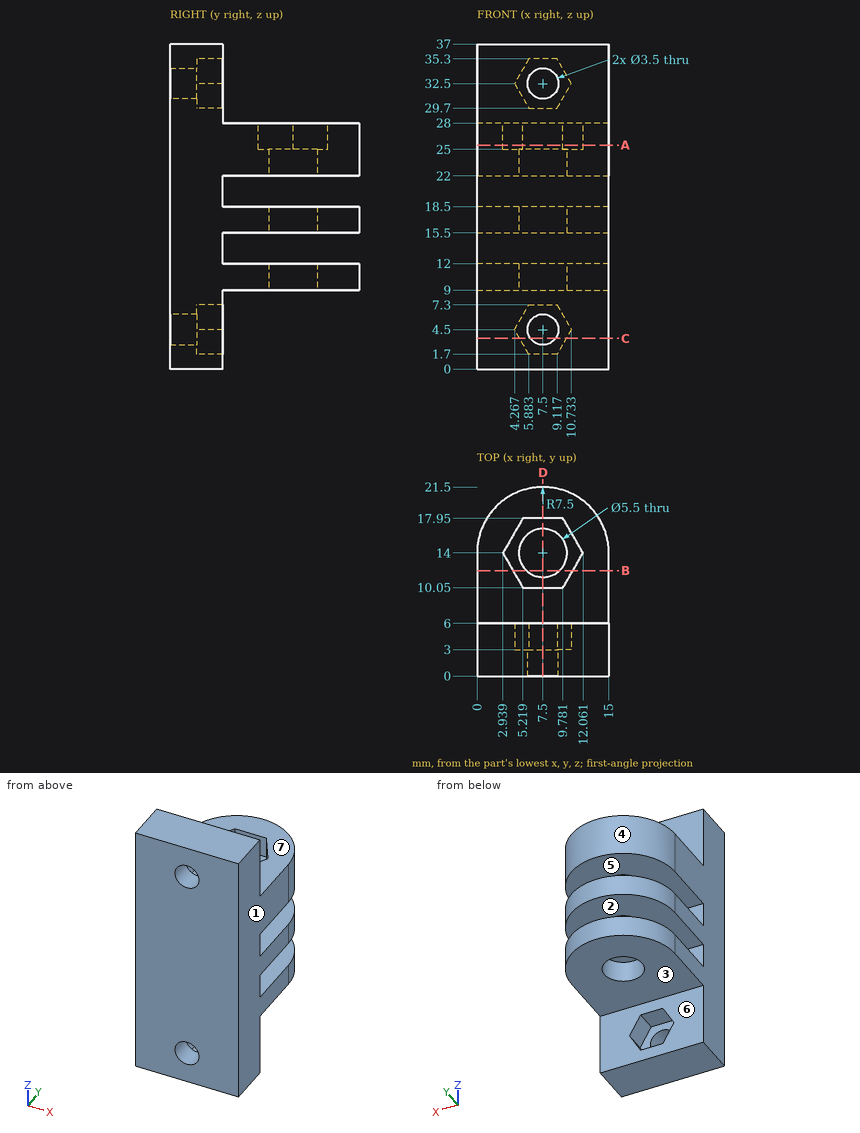
For this review, use the dimensioned drawing (mm, ordinates from the lowest corner) and the shaded views. A direction names the side the tool comes from. Give positions to 0.01 mm unless a question says otherwise; leave off trailing zeros. Write each loop counter-clockwise with the first axis right and the second up, starting at its lowest first coordinate (ties: lowest second). Pieces come first, ordered by that corner, then holes. Notation, with made-up numbers: M -27,1 L 9,1 A13 ccw 9,13 Z; hole C 1,8.25 d10. An arc over 180 degrees is marked long. Answer as a JSON object with one key per item and string values. Group by question number.
1) Mouldability with a two-part tool opening along Z and no side actions: class the marked faces 1, 2 and 3 as released by +Z, released by -Z, zero draft, split by the parting line, or undercut.
2) We need section A-A (z = 25.5). Give the boundary of the cut face in (x, y).
3) Tool access review of the marked faces 4, 5, 6 and 7: name each direction out of +Z, -Z, +X, -X, +Y, -Y from which nothing blocks a thin tool from reaching the whole face with its end or side.
4) We need section B-B (y = 12). Give the boundary of the cut face in (x, z).
5) We need section C-C (z = 3.5). Give the boundary of the cut face in (x, y) (1 decimal).
6) For line 1 along Z through (x, y) = (8.5, 5.75); line 2 along Z through (x, y) = (11.75, 7.25); line 3 along Y through (x, z) = (7.5, 16.6), list the stretches that pass through material, from the lowest coordinate up.
7) We need section D-D (x = 7.5). Count the separate pieces of the cut face and the enclosed holes in it, and give its area (3 significant figures).
8) Clearance check with flat-ended pins moving along their axes: pin 1 Ø9 at (x, y) = (7.5, 14) entering from -Z; pin 2 Ø9 at (x, y) = (7.5, 14) entering from +Z; pin 3 Ø2 at (x, z) = (7.5, 32.5) entering from -Y; pin 4 Ø6 at (x, z) = (13, 10.5) entering from +Y. State where each tip first meets the part, or that it passes through.
Answer key:
{
 "1": {"face 1": "zero draft", "face 2": "undercut", "face 3": "released by -Z"},
 "2": {"outline": "M 0,0 L 15,0 L 15,14 A7.5 ccw 0,14 Z; hole M 2.94,14 L 5.22,10.05 L 9.78,10.05 L 12.06,14 L 9.78,17.95 L 5.22,17.95 Z"},
 "3": {"face 4": "+Z, -Z, +Y", "face 5": "+X, -X, +Y", "face 6": "-Z, +X, -X, +Y", "face 7": "+Z, +X, -X, +Y"},
 "4": {"outline": "M 0,9 L 5.61,9 L 5.61,12 L 0,12 Z; M 0,15.5 L 5.61,15.5 L 5.61,18.5 L 0,18.5 Z; M 0,22 L 5.61,22 L 5.61,25 L 4.09,25 L 4.09,28 L 0,28 Z; M 9.39,9 L 15,9 L 15,12 L 9.39,12 Z; M 9.39,15.5 L 15,15.5 L 15,18.5 L 9.39,18.5 Z; M 9.39,22 L 15,22 L 15,28 L 10.91,28 L 10.91,25 L 9.39,25 Z"},
 "5": {"outline": "M 0,0 L 6.1,0 L 6.1,3 L 4.8,3 L 4.8,6 L 0,6 Z; M 8.9,0 L 15,0 L 15,6 L 10.2,6 L 10.2,3 L 8.9,3 Z"},
 "6": {"line 1": "z = 0 to 1.7, 7.3 to 29.7, 35.3 to 37", "line 2": "z = 9 to 12, 15.5 to 18.5, 22 to 28", "line 3": "y = 0 to 11.25, 16.75 to 21.5"},
 "7": {"separate pieces": "6", "enclosed holes": "0", "area": "280 mm²"},
 "8": {"pin 1": "stops at z = 9", "pin 2": "stops at z = 28", "pin 3": "passes through", "pin 4": "stops at y = 21.07"}
}
